Autodesk Inventor part; units mm, degrees
ref_plane "YZ Plane" through (0, 0, 0) normal (1, 0, 0) x (0, 1, 0)
ref_plane "XZ Plane" through (0, 0, 0) normal (0, 1, 0) x (-1, 0, 0)
ref_plane "XY Plane" through (0, 0, 0) normal (0, 0, 1) x (1, 0, 0)
sketch "Boceto1" plane through (0, 0, 0) normal (0, 1, 0) x (-1, 0, 0)
  line L0 (0, 0) -> (40, 0)
  line L1 (40, 0) -> (40, -100)
  line L2 (40, -100) -> (0, -100)
  line L3 (0, -100) -> (0, 0)
  circle A0 centre (19.95, -16.5) radius 1.5
  circle A1 centre (4, -16.5) radius 1.5
  circle A2 centre (19.95, -83.5) radius 1.5
  circle A3 centre (4, -83.5) radius 1.5
  point P0 (20, 0)
  dimension "d0" = 40
  dimension "d1" = 100
  dimension "d2" = 3
  dimension "d3" = 3
  dimension "d4" = 3
  dimension "d5" = 3
  dimension "d6" = 16.5
  dimension "d7" = 4
  dimension "d8" = 15.95
  dimension "d9" = 16.5
  dimension "d10" = 16.5
  dimension "d11" = 16.5
  dimension "d12" = 4
  dimension "d13" = 15.95
extrude "Extrusión1" add sketch "Boceto1" along normal blind 5
sketch "Boceto2" plane through (0, 5, 0) normal (0, 1, 0) x (1, 0, 0)
  circle A0 centre (-2.5, 2.5) radius 1.5
  line L0 (0, 0) -> (0, 100)
  line L1 (-40, 0) -> (0, 0)
  circle A1 centre (-2.5, 97.5) radius 1.5
  line L2 (0, 100) -> (-40, 100)
  dimension "d16" = 3
  dimension "d17" = 2.5
  dimension "d18" = 2.5
  dimension "d19" = 3
  dimension "d20" = 2.5
  dimension "d21" = 2.5
extrude "Extrusión2" cut sketch "Boceto2" against normal blind 5
sketch "Boceto3" plane through (0, 5, 0) normal (0, 1, 0) x (1, 0, 0)
  line L0 (-40, 0) -> (0, 0)
  line L1 (-14.618, 24) -> (-8, 24)
  line L2 (-8, 24) -> (-8, 9)
  line L3 (-8, 9) -> (-14.618, 9)
  line L4 (-14.618, 9) -> (-14.618, 24)
  line L5 (0, 0) -> (0, 100)
  line L6 (-14.618, 91) -> (-8, 91)
  line L7 (-8, 91) -> (-8, 76)
  line L8 (-8, 76) -> (-14.618, 76)
  line L9 (-14.618, 76) -> (-14.618, 91)
  line L10 (0, 100) -> (-40, 100)
  dimension "d33" = 15
  dimension "d34" = 6.618
  dimension "d35" = 9
  dimension "d36" = 8
  dimension "d37" = 15
  dimension "d38" = 6.618
  dimension "d39" = 8
  dimension "d40" = 9
sketch "Boceto4" plane through (0, 5, 0) normal (0, 1, 0) x (1, 0, 0)
  point P0 (0, 0)
extrude "Extrusión3" cut sketch "Boceto3" against normal blind 0.5
sketch "Boceto5" plane through (0, 5, 0) normal (0, 1, 0) x (1, 0, 0)
  circle A0 centre (-19.95, 16.5) radius 1.5
  circle A1 centre (-19.95, 16.5) radius 1.5
  circle A2 centre (-4, 16.5) radius 1.5
  circle A3 centre (-4, 16.5) radius 1.5
  circle A4 centre (-19.95, 83.5) radius 1.5
  circle A5 centre (-19.95, 83.5) radius 1.5
  circle A6 centre (-4, 83.5) radius 1.5
  circle A7 centre (-4, 83.5) radius 1.5
  point P0 (0, 0)
extrude "Extrusión4" add sketch "Boceto5" against normal blind 5
sketch "Boceto6" plane through (0, 5, 0) normal (0, 1, 0) x (1, 0, 0)
  line L0 (-8, 24) -> (-8, 9)
  line L1 (-8, 9) -> (-8, 16.5)
  line L2 (-8, 16.5) -> (-8, 19.5)
  line L3 (-14.618, 9) -> (-14.618, 24)
  line L4 (-14.618, 9) -> (-14.618, 16.5)
  circle A0 centre (-4, 16.5) radius 1.25
  circle A1 centre (-18.618, 16.5) radius 1.25
  circle A2 centre (-4, 83.5) radius 1.25
  circle A3 centre (-18.618, 83.5) radius 1.25
  line L5 (-8, 91) -> (-8, 76)
  line L6 (-14.618, 76) -> (-14.618, 91)
  line L7 (-14.618, 91) -> (-8, 91)
  point P0 (0, 0)
  dimension "d45" = 7.5
  dimension "d49" = 2.5
  dimension "d50" = 2.5
  dimension "d51" = 4
  dimension "d52" = 4
  dimension "d53" = 2.5
  dimension "d54" = 2.5
  dimension "d55" = 4
  dimension "d56" = 4
  dimension "d57" = 7.5
  dimension "d58" = 7.5
extrude "Extrusión5" cut sketch "Boceto6" against normal blind 5
sketch "Boceto7" plane through (0, 5, 0) normal (0, 1, 0) x (1, 0, 0)
  circle A0 centre (-18.618, 16.5) radius 1.25
  circle A1 centre (-18.618, 16.5) radius 1.25
  circle A2 centre (-4, 16.5) radius 1.25
  circle A3 centre (-4, 16.5) radius 1.25
  circle A4 centre (-18.618, 83.5) radius 1.25
  circle A5 centre (-18.618, 83.5) radius 1.25
  circle A6 centre (-4, 83.5) radius 1.25
  circle A7 centre (-4, 83.5) radius 1.25
  point P0 (0, 0)
extrude "Extrusión6" add sketch "Boceto7" against normal blind 5
sketch "Boceto8" plane through (0, 5, 0) normal (0, 1, 0) x (1, 0, 0)
  circle A0 centre (-20.618, 16.5) radius 1.25
  circle A1 centre (-2, 16.5) radius 1.25
  line L0 (-8, 24) -> (-8, 9)
  line L1 (-14.618, 9) -> (-14.618, 24)
  line L2 (-8, 9) -> (-14.618, 9)
  circle A2 centre (-2, 83.5) radius 1.25
  circle A3 centre (-20.618, 83.5) radius 1.25
  line L3 (-14.618, 91) -> (-8, 91)
  line L4 (-8, 91) -> (-8, 76)
  line L5 (-14.618, 76) -> (-14.618, 91)
  point P0 (0, 0)
  point P1 (-8, 83.5)
  dimension "d63" = 2.5
  dimension "d64" = 2.5
  dimension "d65" = 6
  dimension "d66" = 6
  dimension "d67" = 7.5
  dimension "d68" = 7.5
  dimension "d69" = 2.5
  dimension "d70" = 2.5
  dimension "d71" = 7.5
  dimension "d72" = 7.5
  dimension "d73" = 6
  dimension "d74" = 6
extrude "Extrusión7" cut sketch "Boceto8" against normal blind 6
sketch "Boceto9" plane through (0, 5, 0) normal (0, 1, 0) x (1, 0, 0)
  line L0 (-14.618, 9) -> (-14.618, 24)
  line L1 (-8, 24) -> (-8, 9)
  line L2 (-14.618, 24) -> (-8, 24)
  line L3 (-8, 24) -> (-8, 9)
  line L4 (-8, 9) -> (-14.618, 9)
  line L5 (-14.618, 9) -> (-14.618, 24)
  line L6 (-14.618, 91) -> (-8, 91)
  line L7 (-8, 76) -> (-14.618, 76)
  line L8 (-14.618, 91) -> (-8, 91)
  line L9 (-8, 91) -> (-8, 76)
  line L10 (-8, 76) -> (-14.618, 76)
  line L11 (-14.618, 76) -> (-14.618, 91)
  line L12 (-8, 91) -> (-8, 76)
  line L13 (-14.618, 91) -> (-8, 91)
  line L14 (-8, 91) -> (-8, 76)
  line L15 (-8, 76) -> (-14.618, 76)
  line L16 (-14.618, 76) -> (-14.618, 91)
  line L17 (-14.618, 24) -> (-8, 24)
  line L18 (-8, 24) -> (-8, 9)
  line L19 (-8, 9) -> (-14.618, 9)
  line L20 (-14.618, 9) -> (-14.618, 24)
  point P0 (0, 0)
extrude "Extrusión8" add sketch "Boceto9" against normal blind 0.5
sketch "Boceto10" plane through (0, 5, 0) normal (0, 1, 0) x (1, 0, 0)
  circle A0 centre (-2, 16.5) radius 1.25
  circle A1 centre (-2, 16.5) radius 1.25
  circle A2 centre (-4.691, 16.5) radius 1.25
  circle A3 centre (-23.309, 16.5) radius 1.25
  circle A4 centre (-20.618, 16.5) radius 1.25
  circle A5 centre (-4.691, 83.5) radius 1.25
  circle A6 centre (-23.309, 83.5) radius 1.25
  circle A7 centre (-2, 83.5) radius 1.25
  circle A8 centre (-20.618, 83.5) radius 1.25
  point P0 (0, 0)
  dimension "d79" = 2.5
  dimension "d80" = 2.691
  dimension "d81" = 2.5
  dimension "d82" = 2.691
  dimension "d83" = 2.5
  dimension "d84" = 2.5
  dimension "d85" = 2.691
  dimension "d86" = 2.691
extrude "Extrusión9" cut sketch "Boceto10" against normal blind 5 contours A2 | A3 | A5 | A6
sketch "Boceto11" plane through (0, 5, 0) normal (0, 1, 0) x (1, 0, 0)
  circle A0 centre (-20.618, 16.5) radius 1.25
  circle A1 centre (-20.618, 16.5) radius 1.25
  circle A2 centre (-2, 16.5) radius 1.25
  circle A3 centre (-2, 16.5) radius 1.25
  circle A4 centre (-20.618, 83.5) radius 1.25
  circle A5 centre (-20.618, 83.5) radius 1.25
  circle A6 centre (-2, 83.5) radius 1.25
  circle A7 centre (-2, 83.5) radius 1.25
  point P0 (0, 0)
extrude "Extrusión10" add sketch "Boceto11" against normal blind 5
sketch "Boceto12" plane through (0, 5, 0) normal (0, 1, 0) x (1, 0, 0)
  circle A0 centre (-36.5, 2.5) radius 1.5
  circle A1 centre (-2.5, 2.5) radius 1.5
  circle A2 centre (-36.5, 97.5) radius 1.5
  circle A3 centre (-2.5, 97.5) radius 1.5
  point P0 (0, 0)
  dimension "d91" = 3
  dimension "d92" = 34
  dimension "d93" = 3
  dimension "d94" = 34
extrude "Extrusión11" cut sketch "Boceto12" against normal blind 10 contours A0 | A2
sketch "Boceto13" plane through (0, 5, 0) normal (0, 1, 0) x (1, 0, 0)
  circle A0 centre (-35.31, 38.04) radius 1.25
  circle A1 centre (-35.32, 61.96) radius 1.25
  line L0 (-40, 100) -> (-40, 0)
  line L1 (-40, 0) -> (0, 0)
  dimension "d97" = 2.5
  dimension "d98" = 2.5
  dimension "d99" = 23.92
  dimension "d100" = 4.68
  dimension "d101" = 4.69
  dimension "d102" = 38.04
extrude "Extrusión12" cut sketch "Boceto13" against normal blind 10
sketch "Boceto14" plane through (0, 5, 0) normal (0, 1, 0) x (1, 0, 0)
  circle A0 centre (-30.875, 61.96) radius 0.5
  line L0 (-40, 100) -> (-40, 0)
  line L1 (0, 100) -> (-40, 100)
  circle A1 centre (-30.875, 38.04) radius 0.5
  line L2 (-40, 0) -> (0, 0)
  dimension "d105" = 1
  dimension "d106" = 9.125
  dimension "d107" = 38.04
  dimension "d108" = 1
  dimension "d109" = 9.125
  dimension "d110" = 38.04
extrude "Extrusión13" cut sketch "Boceto14" against normal blind 10
sketch "Boceto15" plane through (0, 5, 0) normal (0, 1, 0) x (1, 0, 0)
  circle A0 centre (-35.31, 38.04) radius 1.25
  circle A1 centre (-35.31, 38.04) radius 1.25
  circle A2 centre (-35.32, 61.96) radius 1.25
  circle A3 centre (-35.32, 61.96) radius 1.25
  point P0 (0, 0)
extrude "Extrusión14" add sketch "Boceto15" against normal blind 10
equation "\"d75\" = d73"
properties part number "Base"
Read the model definition and answer for the solid it produces. Units are mm, in the model's axes. A direction names the side the tool comes from. Give positions to 0.01 mm unless a question says otherwise; leave off trailing zeros. Loops run counter-clockwise (first coordinate to the right, second up) from the corner with the lowest first, then second, coordinate; pieces in that order, holes last.
Item 1: The part is cut by section B-B (x = -2.5). Write down the section's boundary in (y, z).
Item 2: Find the intervals of material crossed by line 1 along X through (y, z) = (3.85, -2.5); line 2 along X through (y, z) = (2.5, -16.5); line 3 along Z through (x, y) = (-36.5, 1.3), in increasing order.
Item 3: The part is cut by section D-D (z = -57). Write down the section's boundary in (x, y).
Item 4: For faces 5 (the cylindrical face through (-34.12, -2.46, -38.42)), 6 (the cylindrical face through (-37.7, 2.5, -1.6)), determine the directions among +Z, -Z, +X, -X, +Y, -Y from which every point of the face is accessible in a straight line to the end or side of a thin tool.
Item 5: The mould has two halves that part along X. Classify faces 1 (the cylindrical face through (-35.59, -2.46, -60.74)), 2 (the cylindrical face through (-4.019, 2.535, -17.554)), 3 (the flat face through (-20, 2, -100)), 4 (the cylindrical face through (-2.695, 2.535, -98.987)): released by +X, released by -X, zero draft, split by the parting line, or undercut.
Item 6: This flat-tipped pin is pushed along its axis until it touches: pin 1 Ø3.5 at (x, z) = (-36.5, -2.5) entering from -Y. Where does it stop, or does it pass through?
Item 7: The part is cut by section C-C (y = -2). Write down the section's boundary in (x, z), and give its area (3 significant figures).
Item 8: The part is cut by section A-A (z = -83.5). Write down the section's boundary in (x, y).
Taken from the geometry:
1. outline: (0, -100) - (5, -100) - (5, -99) - (0, -99) - close; (0, -96) - (5, -96) - (5, -4) - (0, -4) - close; (0, -1) - (5, -1) - (5, 0) - (0, 0) - close
2. line 1: x = -40 to -38, -35 to -4, -1 to 0
2. line 2: x = -40 to -24.56, -22.06 to -5.94, -3.44 to 0
2. line 3: z = -100 to -99, -96 to -4, -1 to 0
3. outline: (-40, 0) - (0, 0) - (0, 5) - (-40, 5) - close
4. face 5: -Y
4. face 6: +Y, -Y
5. face 1: split by the parting line
5. face 2: undercut
5. face 3: zero draft
5. face 4: undercut
6. pin 1: stops at y = 0
7. outline: circle Ø2.5 at (-35.32, -61.96); circle Ø2.5 at (-35.31, -38.04)
7. area: 9.82 mm2
8. outline: (-40, 0) - (-24.56, 0) - (-24.56, 5) - (-40, 5) - close; (-22.06, 0) - (-5.94, 0) - (-5.94, 5) - (-22.06, 5) - close; (-3.44, 0) - (0, 0) - (0, 5) - (-3.44, 5) - close
